```python
from build123d import *

# Parameters (mm, degrees)
SKETCH1_R                      = 6.1
THICKNESS_DEPTH                = 3.5
BOTNUTCUT_START                = -2
SKETCH2_R                      = 2.85
BOTNUTCUT_DEPTH                = 2.6
SKETCH3_R                      = 1.55
BOTSCREWCUT_DEPTH              = 2
CUT_EXTRUDE1_START             = -7
CUT_EXTRUDE1_DEPTH             = 7
RAILNUTCUT_START               = -2
RAILNUTCUT_DEPTH               = 2.6
SKETCH7_R                      = 1.55
RAILSCREWCUT_DEPTH             = 2.6
RAILSCREWCUT_DIRECTION_2_REACH = 53.909
RAILNUTHEADCUT_REACH           = 56.409
RAILNUTHEADCUT_START           = -2.5
SKETCH8_R                      = 2.85
SKETCH9_W                      = 7
SKETCH9_H                      = 0.5
MOVEMENTCUT_DEPTH              = 7
SKETCH10_R                     = 4.5
BOSS_EXTRUDE1_DEPTH            = 3.5
CUT_EXTRUDE2_START             = -50
SKETCH11_W                     = 40
SKETCH11_H                     = 25
CUT_EXTRUDE2_DEPTH             = 25


with BuildPart() as part:
    # Sketch1 → Thickness (new, symmetric)
    with BuildSketch(Plane.XY):
        with BuildLine():
            Line((-13, -50), (13, -50))
            Line((13, -50), (8.424323952, -3.441041405))
            ThreePointArc((8.424323952, -3.441041405), (0, 9.1), (-8.424323952, -3.441041405))
            Line((-8.424323952, -3.441041405), (-13, -50))
        make_face()
        Circle(SKETCH1_R, mode=Mode.SUBTRACT)
    extrude(amount=THICKNESS_DEPTH, both=True)

    # Sketch2 → BotNutCut (cut)
    with BuildSketch(Plane.XZ.offset(50).offset(BOTNUTCUT_START)):
        with Locations((-7.5, 0)):
            Circle(SKETCH2_R)
        with BuildLine():
            Line((-10.790896534, 2.85), (-10.790896534, 0))
            Line((-10.790896534, 0), (-9.968172361, -1.42500007))
            ThreePointArc((-9.968172361, -1.42500007), (-9.96817242, 1.424999968), (-7.499999995, 2.85))
            Line((-7.499999995, 2.85), (-10.790896534, 2.85))
        make_face()
        with BuildLine():
            Line((-4.209103466, 2.85), (-7.499999995, 2.85))
            ThreePointArc((-7.499999995, 2.85), (-5.484745672, 2.015254324), (-4.65, 0))
            ThreePointArc((-4.65, 0), (-4.747111384, -0.737634237), (-5.031827556, -1.424999925))
            Line((-5.031827556, -1.424999925), (-4.209103466, 0))
            Line((-4.209103466, 0), (-4.209103466, 2.85))
        make_face()
        with BuildLine():
            ThreePointArc((-5.031827556, -1.424999925), (-6.074999963, -2.468172379), (-7.5, -2.85))
            Line((-7.5, -2.85), (-5.854551733, -2.85))
            Line((-5.854551733, -2.85), (-5.031827556, -1.424999925))
        make_face()
        with BuildLine():
            ThreePointArc((-7.5, -2.85), (-8.924999965, -2.468172421), (-9.968172361, -1.42500007))
            Line((-9.968172361, -1.42500007), (-9.145448267, -2.85))
            Line((-9.145448267, -2.85), (-7.5, -2.85))
        make_face()
        with BuildLine():
            ThreePointArc((7.5, -2.85), (6.074999995, -2.468172398), (5.031827593, -1.42499999))
            Line((5.031827593, -1.42499999), (5.854551733, -2.85))
            Line((5.854551733, -2.85), (7.5, -2.85))
        make_face()
        with BuildLine():
            ThreePointArc((9.968172375, -1.425000045), (8.924999978, -2.468172414), (7.5, -2.85))
            Line((7.5, -2.85), (9.145448267, -2.85))
            Line((9.145448267, -2.85), (9.968172375, -1.425000045))
        make_face()
        with BuildLine():
            Line((10.790896534, 2.85), (7.5, 2.85))
            ThreePointArc((7.5, 2.85), (9.515254326, 2.015254326), (10.35, 0))
            ThreePointArc((10.35, 0), (10.252888598, -0.737634304), (9.968172375, -1.425000045))
            Line((9.968172375, -1.425000045), (10.790896534, 0))
            Line((10.790896534, 0), (10.790896534, 2.85))
        make_face()
        with BuildLine():
            Line((4.209103466, 2.85), (4.209103466, 0))
            Line((4.209103466, 0), (5.031827593, -1.42499999))
            ThreePointArc((5.031827593, -1.42499999), (5.031827602, 1.425000005), (7.5, 2.85))
            Line((7.5, 2.85), (4.209103466, 2.85))
        make_face()
        with Locations((7.5, 0)):
            Circle(SKETCH2_R)
    extrude(amount=-BOTNUTCUT_DEPTH, mode=Mode.SUBTRACT)

    # Sketch3 → BotScrewCut (cut)
    with BuildSketch(Plane.XZ.offset(50)):
        with Locations(Location((-7.5, 0, 0), (0, 0, 270))):
            Circle(SKETCH3_R)
        with Locations(Location((7.5, 0, 0), (0, 0, 270))):
            Circle(SKETCH3_R)
    extrude(amount=-BOTSCREWCUT_DEPTH, mode=Mode.SUBTRACT)

    # Sketch5 → Cut-Extrude1 (cut)
    with BuildSketch(Plane.XY.offset(3.5).offset(CUT_EXTRUDE1_START)):
        with BuildLine():
            ThreePointArc((0.5, -6.079473661), (0, -6.1), (-0.5, -6.079473661))
            Line((-0.5, -6.079473661), (-0.5, -12.924568984))
            ThreePointArc((-0.5, -12.924568984), (0, -23.1), (0.5, -12.924568984))
            Line((0.5, -12.924568984), (0.5, -6.079473661))
        make_face()
    extrude(amount=CUT_EXTRUDE1_DEPTH, mode=Mode.SUBTRACT)

    # Sketch6 → RailNutCut (cut)
    with BuildSketch(Plane(origin=(-0.5, 0, 0), x_dir=(0, 0, -1), z_dir=(1, 0, 0)).offset(RAILNUTCUT_START)):
        Polygon((0, -13.290896534), (2.85, -11.645448267), (2.85, -8.354551733), (0, -6.709103466), (-2.85, -6.709103466), (-2.85, -13.290896534), align=None)
    extrude(amount=-RAILNUTCUT_DEPTH, mode=Mode.SUBTRACT)

    # Sketch7 → RailScrewCut (cut)
    with BuildSketch(Plane(origin=(-0.5, 0, 0), x_dir=(0, 0, -1), z_dir=(1, 0, 0))):
        with Locations(Location((0, -10, 0), (0, 0, 270))):
            Circle(SKETCH7_R)
    extrude(amount=-RAILSCREWCUT_DEPTH, mode=Mode.SUBTRACT)

    # RailScrewCut direction 2: up to this plane
    railscrewcut_direction_2_end = Plane(origin=(13, -50, 3.5), z_dir=(-0.9952055153223801, -0.09780583966162733, 0))
    # Sketch7 → RailScrewCut direction 2 (cut, up to the surface)
    with BuildSketch(Plane(origin=(-0.5, 0, 0), x_dir=(0, 0, -1), z_dir=(1, 0, 0)), mode=Mode.PRIVATE) as railscrewcut_direction_2_sk1:
        with Locations(Location((0, -10, 0), (0, 0, 270))):
            Circle(SKETCH7_R)
    railscrewcut_direction_2_tool1 = split(extrude(railscrewcut_direction_2_sk1.sketch, amount=RAILSCREWCUT_DIRECTION_2_REACH, mode=Mode.PRIVATE), bisect_by=railscrewcut_direction_2_end, keep=Keep.BOTH, mode=Mode.PRIVATE)
    add(railscrewcut_direction_2_tool1.solids().sort_by_distance((-0.5, -10, 0))[0], mode=Mode.SUBTRACT)

    # RailNutHeadCut: up to this plane
    railnutheadcut_end = Plane(origin=(13, -50, 3.5), z_dir=(-0.9952055153223801, -0.09780583966162733, 0))
    # Sketch8 → RailNutHeadCut (cut, up to the surface)
    with BuildSketch(Plane.ZY.offset(-0.5).offset(RAILNUTHEADCUT_START), mode=Mode.PRIVATE) as railnutheadcut_sk1:
        with Locations(Location((0, -10, 0), (0, 0, 270))):
            Circle(SKETCH8_R)
    railnutheadcut_tool1 = split(extrude(railnutheadcut_sk1.sketch, amount=-RAILNUTHEADCUT_REACH, mode=Mode.PRIVATE), bisect_by=railnutheadcut_end, keep=Keep.BOTH, mode=Mode.PRIVATE)
    add(railnutheadcut_tool1.solids().sort_by_distance((3, -10, 0))[0], mode=Mode.SUBTRACT)

    # Sketch9 → MovementCut (cut)
    with BuildSketch(Plane.XY.offset(3.5)):
        with Locations((7.5, -18.75)):
            Rectangle(SKETCH9_W, SKETCH9_H)
    extrude(amount=-MOVEMENTCUT_DEPTH, mode=Mode.SUBTRACT)

    # Sketch10 → Boss-Extrude1 (add, symmetric)
    with BuildSketch(Plane.XY):
        with BuildLine():
            Line((-0.5, -13.527864045), (-0.5, -12.924568984))
            ThreePointArc((-0.5, -12.924568984), (-3.780537731, -21.42308844), (5.0009999, -19))
            Line((5.0009999, -19), (4.387482194, -19))
            ThreePointArc((4.387482194, -19), (-3.356217727, -20.997632828), (-0.5, -13.527864045))
        make_face()
        with Locations((0, -18)):
            Circle(SKETCH10_R)
    extrude(amount=BOSS_EXTRUDE1_DEPTH, both=True)

    # Sketch11 → Cut-Extrude2 (cut)
    with BuildSketch(Plane(origin=(0, 0, 0), x_dir=(1, 0, 0), z_dir=(0, 1, 0)).offset(CUT_EXTRUDE2_START)):
        Rectangle(SKETCH11_W, SKETCH11_H)
    extrude(amount=CUT_EXTRUDE2_DEPTH, mode=Mode.SUBTRACT)


solid = part.part
```
Work out the finished part from the listing and answer in its coordinate system (mm). A direction names the side the tool comes from. Give positions to 0.01 mm unless a question says otherwise; leave off trailing zeros. Loops run counter-clockwise (first coordinate to the right, second up) from the corner with the lowest first, then second, coordinate; pieces in that order, holes last. Notation, with made-up numbers: (-4, 20) -> (35, 20) arc R21 cw to (35, 51) -> close; hole circle Ø7 at (56, -22). An arc over 180 degrees is marked (long way). Write item = value, one per line. Start each with the question number.
(1) The mould has two halves that part along X. Classify faces 4 (the cylindrical face through (-1.49, -8.77, 0.94)), 5 (the flat face through (-0.5, -10, 2)), 6 (the flat face through (-9.47, -14.07, 0.05)): +X half, -X half, draft (parallel to the pull), parting line (faces both ways), or undercut.
(2) Find section B-B on y = 0. Give the vertices of the cut face in (x, z), and give its area (3 significant figures).
(3) Which of the six approach directions +Z, -Z, +X, -X, +Y, -Y give full straight-line access (tool end or side, diameter ignored) to faces 1 (the flat face through (-3.782, -12.48, -1.405)), 2 (the flat face through (10.252, -22.042, 0.049)), 3 (the flat face through (9.34, -12.75, 1.6))?
(4) Find section D-D on x = 0. Give the vertices of the cut face in (y, z).
(5) Given pin 1 Ø3 at (x, z) = (-4, 1) entering from +Y; pin 2 Ø3 at (y, z) = (-10, 0) entering from -X; pin 3 Ø1.5 at (y, z) = (2.5, -1.5) entering from +X, each flat-ended and moving along its own axis, determine where each tip first touches the part or whether it passes through.
(6) Find section C-C on x = 8.75. Give the vertices of the cut face in (y, z), and give its area (3 significant figures).
(7) Find the intervals of material crossed by probe 1 along Y at (x, z) = (0, 1.5); probe 2 along X at (y, z) = (0, 0.5); probe 3 along Y at (x, z) = (4, -0.75), in increasing order. Write a range as from..to.
(8) Find section A-A on y = -12. Give the vertices of the cut face in (x, z), and give its area (3 significant figures).
From the geometry:
q1.face_4 = draft
q1.face_5 = undercut
q1.face_6 = -X half
q2.outline = (-9.1, -3.5) -> (-6.1, -3.5) -> (-6.1, 3.5) -> (-9.1, 3.5) -> close; (6.1, -3.5) -> (9.1, -3.5) -> (9.1, 3.5) -> (6.1, 3.5) -> close
q2.area = 42.0 mm^2
q3.face_1 = none
q3.face_2 = +Z, -Z, +X, +Y
q3.face_3 = +Z, -Z, +X
q4.outline = (-25, -3.5) -> (-13.5, -3.5) -> (-13.5, 3.5) -> (-25, 3.5) -> close; (6.1, -3.5) -> (9.1, -3.5) -> (9.1, 3.5) -> (6.1, 3.5) -> close
q5.pin_1 = 8.75
q5.pin_2 = -9.22
q5.pin_3 = 8.93
q6.outline = (-25, -3.5) -> (-19, -3.5) -> (-19, 3.5) -> (-25, 3.5) -> close; (-18.5, -3.5) -> (-6.75, -3.5) -> (-6.75, 3.5) -> (-18.5, 3.5) -> close; (-2.5, -3.5) -> (2.5, -3.5) -> (2.5, 3.5) -> (-2.5, 3.5) -> close; hole circle Ø5.7 at (-10, 0)
q6.area = 134 mm^2
q7.probe_1 = -25..-13.5, 6.1..9.1
q7.probe_2 = -9.1..-6.1, 6.1..9.1
q7.probe_3 = -25..-15.94, -14.84..-12.75, -7.25..-4.61, 4.61..8.17
q8.outline = (-9.27, -3.5) -> (-0.5, -3.5) -> (-0.5, 3.5) -> (-9.27, 3.5) -> close; (0.5, -3.5) -> (9.27, -3.5) -> (9.27, -2.03) -> (3, -2.03) -> (3, 2.03) -> (9.27, 2.03) -> (9.27, 3.5) -> (0.5, 3.5) -> close; hole (-5.1, -2.24) -> (-2.5, -2.24) -> (-2.5, 2.85) -> (-5.1, 2.85) -> close
q8.area = 84.1 mm^2
